```python
from build123d import *

# Parameters (mm, degrees)
CROQUIS2_R              = 1.5875
CROQUIS2_R_2            = 1.720307827
SALIENTE_EXTRUIR1_DEPTH = 5
CROQUIS2_4_W            = 7.146105916
CROQUIS2_4_H            = 2
SALIENTE_EXTRUIR2_DEPTH = 11
SALIENTE_EXTRUIR3_START = -11
CROQUIS2_5_R            = 1.5875
CROQUIS2_5_R_2          = 1.720307827
SALIENTE_EXTRUIR3_DEPTH = 5


with BuildPart() as part:
    # Croquis2 → Saliente-Extruir1 (new body)
    with BuildSketch(Plane(origin=(0, 0, 0), x_dir=(1, 0, 0), z_dir=(0, 1, 0))):
        with BuildLine():
            ThreePointArc((46.426947042, 35), (49.564233927, 30.472202028), (53.685223181, 34.127468235))
            Line((53.685223181, 34.127468235), (53.573052958, 46.021630377))
            Line((53.573052958, 46.021630377), (53.573052958, 49.021630377))
            Line((53.573052958, 49.021630377), (46.426947042, 49.021630377))
            Line((46.426947042, 49.021630377), (46.426947042, 35))
        make_face()
        with Locations(Location((50.003640725, 34.127468235, 0), (0, 0, 270))):
            Circle(CROQUIS2_R, mode=Mode.SUBTRACT)
        with Locations(Location((50, 43.030352088, 0), (0, 0, 270))):
            Circle(CROQUIS2_R_2, mode=Mode.SUBTRACT)
    extrude(amount=-SALIENTE_EXTRUIR1_DEPTH)

    # Croquis2_4 → Saliente-Extruir2 (add)
    with BuildSketch(Plane(origin=(0, 0, 0), x_dir=(1, 0, 0), z_dir=(0, 1, 0))):
        with Locations((50, 50.021630377)):
            Rectangle(CROQUIS2_4_W, CROQUIS2_4_H)
    extrude(amount=-SALIENTE_EXTRUIR2_DEPTH)

    # Croquis2_5 → Saliente-Extruir3 (add)
    with BuildSketch(Plane(origin=(0, 0, 0), x_dir=(1, 0, 0), z_dir=(0, 1, 0)).offset(SALIENTE_EXTRUIR3_START)):
        with BuildLine():
            ThreePointArc((46.426947042, 35), (49.564233927, 30.472202028), (53.685223181, 34.127468235))
            Line((53.685223181, 34.127468235), (53.573052958, 46.021630377))
            Line((53.573052958, 46.021630377), (53.573052958, 51.021630377))
            Line((53.573052958, 51.021630377), (46.426947042, 51.021630377))
            Line((46.426947042, 51.021630377), (46.426947042, 35))
        make_face()
        with Locations(Location((50.003640725, 34.127468235, 0), (0, 0, 270))):
            Circle(CROQUIS2_5_R, mode=Mode.SUBTRACT)
        with Locations(Location((50, 43.030352088, 0), (0, 0, 270))):
            Circle(CROQUIS2_5_R_2, mode=Mode.SUBTRACT)
    extrude(amount=-SALIENTE_EXTRUIR3_DEPTH)


solid = part.part
```
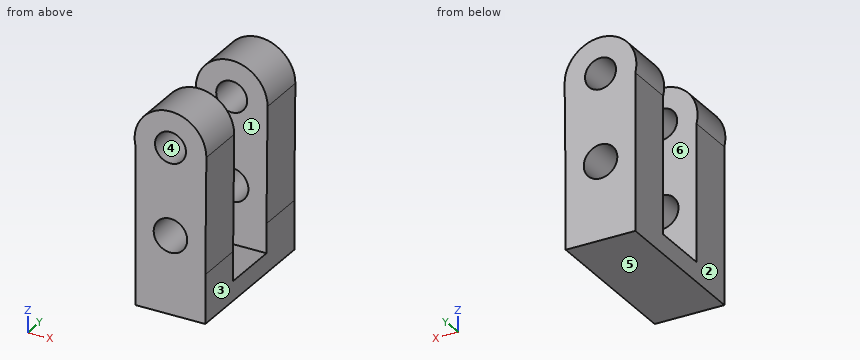
For this review, take the finished solid that the model builds, in its own axes (mm). Face numbers are marked on the shaded views. A direction names the side the tool comes from. Coordinates: 2 decimals unless noted, no trailing zeros. Write each loop counter-clockwise with the first axis right and the second up, starting at its lowest first coordinate (ties: lowest second). Pieces come first, ordered by that corner, then holes. Notation, with made-up numbers: (65.25, -11.75) - (102.25, -11.75) arc R3 cw to (102.25, -7.75) - close; hole circle Ø11 at (31.5, 0). An arc over 180 degrees is marked (long way). Answer in a Markdown table with one row per item. Add a question column.
Q1. We need section A-A, the plane z = -48. State the section outline as (x, y) points.
Q2. For P1, Ø3, axis at x = 50, z = -43.03, coming from the -Y side; P2, Ø1.5, axis at y = -10, z = -48.5, coming from the +X side, all flat-tipped, find the tip position at first contact; note any pin that passes through.
Q3. We need section D-D, the plane y = -8.25. State the section outline as (x, z) points.
Q4. We need section C-C, the plane z = -34.5. State the section outline as (x, y) points, and give its area (3 significant figures).
Q5. For probe 1 along Y at (x, z) = (51, -40.5); probe 2 along Z at (x, y) = (50.5, -12.5); probe 3 along Z at (x, y) = (49.75, -2.75), list the stretches that pass through material, from the lowest coordinate up.
Q6. Draft analysis for pull direction Z (two halves, no side actions). For the marked faces 4, 5 and 6, state which applies: +Z half, -Z half, draft (parallel to the pull), parting line (faces both ways), or undercut.
Q7. Tool access review of the marked faces 1, 2 and 3: name each direction out of +Z, -Z, +X, -X, +Y, -Y from which nothing blocks a thin tool from reaching the whole face with its end or side.
Q8. We need section B-B, the plane x = 51. State the section outline as (y, z) points, and give its area (3 significant figures).
Answer list:
| question | item | result |
|---|---|---|
| 1 | outline | (46.43, -16) - (53.57, -16) - (53.57, -11) - (46.43, -11) - close; (46.43, -5) - (53.57, -5) - (53.57, 0) - (46.43, 0) - close |
| 2 | P1 | passes through |
| 2 | P2 | stops at x = 53.57 |
| 3 | outline | (46.43, -51.02) - (53.57, -51.02) - (53.57, -49.02) - (46.43, -49.02) - close |
| 4 | outline | (46.34, -16) - (48.46, -16) - (48.46, -11) - (46.34, -11) - close; (46.34, -5) - (48.46, -5) - (48.46, 0) - (46.34, 0) - close; (51.55, -16) - (53.68, -16) - (53.68, -11) - (51.55, -11) - close; (51.55, -5) - (53.68, -5) - (53.68, 0) - (51.55, 0) - close |
| 4 | area | 42.5 mm2 |
| 5 | probe 1 | y = -16 to -11, -5 to 0 |
| 5 | probe 2 | z = -51.02 to -44.68, -41.38 to -35.64, -32.62 to -30.48 |
| 5 | probe 3 | z = -51.02 to -44.73, -41.33 to -35.69, -32.56 to -30.45 |
| 6 | face 4 | undercut |
| 6 | face 5 | -Z half |
| 6 | face 6 | draft |
| 7 | face 1 | +Z, +X, -X |
| 7 | face 2 | -Z, -X, +Y, -Y |
| 7 | face 3 | -Z, +X, +Y, -Y |
| 8 | outline | (-16, -51.02) - (0, -51.02) - (0, -44.43) - (-5, -44.43) - (-5, -49.02) - (-11, -49.02) - (-11, -44.43) - (-16, -44.43) - close; (-16, -41.63) - (-11, -41.63) - (-11, -35.36) - (-16, -35.36) - close; (-16, -32.89) - (-11, -32.89) - (-11, -30.58) - (-16, -30.58) - close; (-5, -41.63) - (0, -41.63) - (0, -35.36) - (-5, -35.36) - close; (-5, -32.89) - (0, -32.89) - (0, -30.58) - (-5, -30.58) - close |
| 8 | area | 164 mm2 |
